```python
from build123d import *

# Parameters (mm, degrees)
BOSS_EXTRUDE1_DEPTH = 30
SKETCH3_R           = 7.5
CUT_EXTRUDE3_DEPTH  = 76
SKETCH4_W           = 29.345301095
SKETCH4_H           = 36.901717618
SKETCH4_H_2         = 23.098282382
SKETCH4_W_2         = 30
SKETCH4_H_3         = 43.098282382
SKETCH4_H_4         = 16.901717618
BOSS_EXTRUDE2_DEPTH = 30
SKETCH2_R           = 4.7625
CUT_EXTRUDE2_DEPTH  = 61.901718
SKETCH5_R           = 4.7625
CUT_EXTRUDE4_DEPTH  = 41.901718


with BuildPart() as part:
    # Sketch1 → Boss-Extrude1 (new body)
    with BuildSketch(Plane.XY):
        Polygon((-54, 34.401717618), (54, 34.401717618), (54, -2.5), (24.654698905, -2.5), (24.654698905, -17.5), (54, -17.5), (54, -40.598282382), (-54, -40.598282382), (-54, 2.5), (-24, 2.5), (-24, 17.5), (-54, 17.5), align=None)
    extrude(amount=BOSS_EXTRUDE1_DEPTH)

    # Sketch3 → Cut-Extrude3 (cut, through all)
    with BuildSketch(Plane(origin=(0, 34.401717618, 0), x_dir=(1, 0, 0), z_dir=(0, 1, 0))):
        with Locations((0, -15)):
            Circle(SKETCH3_R)
    extrude(amount=-CUT_EXTRUDE3_DEPTH, mode=Mode.SUBTRACT)

    # Sketch4 → Boss-Extrude2 (add)
    with BuildSketch(Plane(origin=(0, 0, 0), x_dir=(-1, 0, 0), z_dir=(0, 0, -1))):
        with Locations((-39.327349453, 15.950858809)):
            Rectangle(SKETCH4_W, SKETCH4_H)
        with Locations((-39.327349453, -29.049141191)):
            Rectangle(SKETCH4_W, SKETCH4_H_2)
        with Locations((39, -19.049141191)):
            Rectangle(SKETCH4_W_2, SKETCH4_H_3)
        with Locations((39, 25.950858809)):
            Rectangle(SKETCH4_W_2, SKETCH4_H_4)
    extrude(amount=BOSS_EXTRUDE2_DEPTH)

    # Sketch2 → Cut-Extrude2 (cut)
    with BuildSketch(Plane(origin=(0, 34.401717618, 0), x_dir=(1, 0, 0), z_dir=(0, 1, 0))):
        with Locations((39.853186988, 15)):
            Circle(SKETCH2_R)
    extrude(amount=-CUT_EXTRUDE2_DEPTH, mode=Mode.SUBTRACT)

    # Sketch5 → Cut-Extrude4 (cut)
    with BuildSketch(Plane(origin=(0, 34.401717618, 0), x_dir=(1, 0, 0), z_dir=(0, 1, 0))):
        with Locations((-39, 15)):
            Circle(SKETCH5_R)
    extrude(amount=-CUT_EXTRUDE4_DEPTH, mode=Mode.SUBTRACT)


solid = part.part
```
Can you work these out from the model? Positions are in its coordinate system, mm. A direction names the side the tool comes from. Round coordinates to 2 decimals unless told otherwise and drop trailing zeros. Loops run counter-clockwise (first coordinate to the right, second up) from the corner with the lowest first, then second, coordinate; pieces in that order, holes last. Notation, with made-up numbers: (-35, 14.25) -> (-27, 14.25) arc R19 ccw to (-27, 23.25) -> close; hole circle Ø8 at (-28.5, 58). An arc over 180 degrees is marked (long way). One line per item, written item: value. Start each with the question number.
1. If we section it at C-C, the plane x = -39: Write out the boundary of the cut face in (y, z).
2. If we section it at B-B, the plane y = 15: Write out the boundary of the cut face in (x, z) (1 decimal), then the cut area to 3 significant figures.
3. For faces 1 (the flat face through (-39, 26, -30)), 2 (the flat face through (24.655, 16, -15)), 3 (the cylindrical face through (-1.63, -2.57, 22.32)), 4 (the flat face through (24.655, -10, 15)), 5 (the cylindrical face through (36.074, 16.209, -12.102)), which set-ups out of +Z, -Z, +X, -X, +Y, -Y let a thin tool reach every point of the face, with its end or its side?
4. If we mould it in two halves opening along Z, with no side actions, what happens to faces 6 (the flat face through (1, 34.402, 7)), 7 (the flat face through (40, 16, -30)), 8 (the flat face through (-39, -7.5, -15)), 9 (the cylindrical face through (-40.03, 26.07, -10.35))? For each: pulls with the +Z half, pulls with the -Z half, needs draft (parallel to the pull), parting line crosses it, or undercut.
5. If we section it at D-D, the plane z = -21: Write out the boundary of the cut face in (x, y).
6. If we section it at A-A, the plane z = -15: Give the number of separate pieces and of enclosed holes in the cut face, then the cut area to 3 significant figures.
7. For pin 1 (7.5 mm diameter, centred on y = 7, z = 9.5, fed in from -X), with a flat end and sliding along its axis, tell me the tip position at first contact or that it passes through.
8. If I drill on probe 1 along X at (y, z) = (22.5, -15); probe 2 along Y at (x, z) = (-45, 3); probe 3 along X at (y, z) = (20, -11.5), over which ranges is the centre line in solid material (lowest first)?
Calculated:
1. outline: (-40.6, -30) -> (2.5, -30) -> (2.5, -19.76) -> (-7.5, -19.76) -> (-7.5, -10.24) -> (2.5, -10.24) -> (2.5, 30) -> (-40.6, 30) -> close; (17.5, -30) -> (34.4, -30) -> (34.4, -19.76) -> (17.5, -19.76) -> close; (17.5, -10.24) -> (34.4, -10.24) -> (34.4, 30) -> (17.5, 30) -> close
2. outline: (-24, 0) -> (24.7, 0) -> (24.7, -30) -> (54, -30) -> (54, 30) -> (-24, 30) -> close; hole circle Ø15 at (0, 15); hole circle Ø9.5 at (39.9, -15)
2. area: 2,970 mm²
3. face 1: -Z, +X, -X, +Y, -Y
3. face 2: -Z, +Y, -Y
3. face 3: +Y, -Y
3. face 4: +Z, -Z, +X
3. face 5: +Y
4. face 6: needs draft
4. face 7: pulls with the -Z half
4. face 8: undercut
4. face 9: undercut
5. outline: (-54, -40.6) -> (-24, -40.6) -> (-24, 2.5) -> (-54, 2.5) -> close; (-54, 17.5) -> (-24, 17.5) -> (-24, 34.4) -> (-54, 34.4) -> close; (24.65, -40.6) -> (54, -40.6) -> (54, -17.5) -> (24.65, -17.5) -> close; (24.65, -2.5) -> (54, -2.5) -> (54, 34.4) -> (24.65, 34.4) -> close
6. separate pieces: 6
6. enclosed holes: 0
6. area: 2,860 mm²
7. pin 1: stops at x = -24
8. probe 1: x = -54 to -43.76, -34.24 to -24, 24.65 to 35.09, 44.62 to 54
8. probe 2: y = -40.6 to 2.5, 17.5 to 34.4
8. probe 3: x = -54 to -42.23, -35.77 to -24, 24.65 to 36.62, 43.08 to 54
